Read the model definition and answer for the solid it produces. Units are mm, in the model's axes. A direction names the side the tool comes from. Coordinates: 2 decimals unless noted, no trailing zeros. Order: outer loops, then holes, each group sorted by start corner. A loop starts at its lowest first (then second) coordinate and runs counter-clockwise, first axis right, second up. Notation, with made-up numbers: M 30,70.5 L 37,70.5 A11 ccw 37,74.5 Z; hole C 70.5,9.5 d7. An arc over 180 degrees is marked long. Use a Markdown table: item, result. Add a question column.
1) Find section B-B on z = -10. Write down the section's boundary in (x, y).
2) Find the intervals of material crossed by probe 1 along X at (y, z) = (1.5, -32.5); probe 2 along Z at (x, y) = (0, 0.45); probe 3 along Z at (x, y) = (-55.5, 5.75), in increasing order. Write a range as [from, to].
3) For faces 1 (the face through (1, 0, -18)), 2 (the face through (36.007, 2.57, -61.208)), determine the directions among +Z, -Z, +X, -X, +Y, -Y from which every point of the face is accessible in a straight line to the end or side of a thin tool.
4) Find section A-A on y = 9. Write down the section's boundary in (x, z).
5) Each of these flat-tipped pins is pushed along its axis until it touches: pin 1 Ø4 at (x, y) = (50, 4) entering from -Z; pin 2 Ø10 at (x, z) = (-14.5, -5) entering from +Y; pin 3 Ø1.4 at (x, z) = (-56.29, -32.5) entering from -Y; pin 4 Ø5 at (x, y) = (-55.5, 11) entering from +Z. Where does it stop, or does it pass through?
Autodesk Inventor part; units mm, degrees
ref_plane "YZ Plane" through (0, 0, 0) normal (1, 0, 0) x (0, 1, 0)
ref_plane "XZ Plane" through (0, 0, 0) normal (0, 1, 0) x (-1, 0, 0)
ref_plane "XY Plane" through (0, 0, 0) normal (0, 0, 1) x (1, 0, 0)
sketch "Sketch1" plane through (0, 0, 0) normal (0, 1, 0) x (-1, 0, 0)
  line L0 (0, 85) -> (73.6122, 42.5)
  line L1 (73.6122, 42.5) -> (73.6122, -42.5)
  line L2 (73.6122, -42.5) -> (0, -85)
  line L3 (0, -85) -> (-73.6122, -42.5)
  line L4 (-73.6122, -42.5) -> (-73.6122, 42.5)
  line L5 (-73.6122, 42.5) -> (0, 85)
  point P0 (0, 0)
  point P1 (0, 0)
  dimension "d0" = 0
  dimension "d1" = 85
extrude "Extrusion1" add sketch "Sketch1" along normal blind 13
sketch "Sketch2" plane through (0, 13, 0) normal (0, 1, 0) x (1, 0, 0)
  line L0 (0, -82.6906) -> (-71.6122, -41.3453)
  line L1 (-71.6122, -41.3453) -> (-71.6122, 41.3453)
  line L2 (-71.6122, 41.3453) -> (0, 82.6906)
  line L3 (0, 82.6906) -> (71.6122, 41.3453)
  line L4 (71.6122, 41.3453) -> (71.6122, -41.3453)
  line L5 (71.6122, -41.3453) -> (0, -82.6906)
  line L6 (-73.6122, 42.5) -> (-73.6122, -42.5)
  point P0 (0, 0)
  point P1 (0, 0)
  point P2 (0, 0)
  dimension "d6" = 0
  dimension "d7" = 2
extrude "Extrusion2" cut sketch "Sketch2" against normal blind 11
sketch "Sketch3" plane through (0, 2, 0) normal (0, 1, 0) x (1, 0, 0)
  circle A0 centre (0, -65) radius 2
  point P0 (0, 0)
  dimension "d10" = 4
  dimension "d11" = 65
extrude "Extrusion3" add sketch "Sketch3" along normal blind 5
sketch "Sketch4" plane through (0, 7, 65) normal (0, 1, 0) x (1, 0, 0)
  point P0 (0, 65)
  point P1 (0, 0)
  point P2 (0, 0)
  dimension "d14" = 65
  dimension "d15" = 0
hole "Hole1" at (0, 7, 65) direction (0, -1, 0) diameter 1.5 end through all
pattern_circular "Circular Pattern1" count 3 over 360 about axis through (0, -10, 0) along (0, 1, 0) of "Extrusion3", "Hole1"
fillet "Fillet1" radius 2 6 edges at (-71.6122, 2, 0) (-35.8061, 2, 62.0179) (35.8061, 2, 62.0179) (71.6122, 2, 0) (35.8061, 2, -62.0179) (-35.8061, 2, -62.0179)
sketch "Sketch5" plane through (0, 2, 0) normal (0, 1, 0) x (1, 0, 0)
  point P0 (0, 0)
  point P1 (0, 0)
hole "Hole2" at (0, 2, 0) direction (0, -1, 0) diameter 3 depth 3
properties part number "hexlight-top-led-nodule"
Check result:
| question | item | result |
|---|---|---|
| 1 | outline | M -73.61,0 L 73.61,0 L 73.61,13 L 71.61,13 L 71.61,4 A2 cw 69.61,2 L -69.61,2 A2 cw -71.61,4 L -71.61,13 L -73.61,13 Z |
| 2 | probe 1 | x = [-73.61, -57.04], [-55.54, 55.54], [57.04, 73.61] |
| 2 | probe 2 | z = [-85, -1.5], [1.5, 64.25], [65.75, 85] |
| 2 | probe 3 | z = [-52.96, -50.65], [-34.34, -30.66], [50.65, 52.96] |
| 3 | face 1 | +Z, -Z, +X, -X, -Y |
| 3 | face 2 | +Y |
| 4 | outline | M -73.61,-42.5 L 0,-85 L 73.61,-42.5 L 73.61,42.5 L 0,85 L -73.61,42.5 Z; hole M -71.61,-41.35 L 0,-82.69 L 71.61,-41.35 L 71.61,41.35 L 0,82.69 L -71.61,41.35 Z |
| 5 | pin 1 | stops at z = -57.29 |
| 5 | pin 2 | stops at y = 2 |
| 5 | pin 3 | passes through |
| 5 | pin 4 | stops at z = 54.4 |
